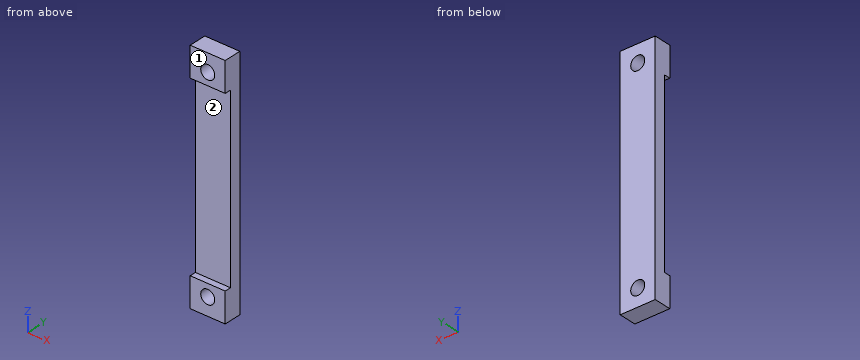
Autodesk Inventor part; units mm, degrees
ref_plane "YZ Plane" through (0, 0, 0) normal (1, 0, 0) x (0, 1, 0)
ref_plane "XZ Plane" through (0, 0, 0) normal (0, 1, 0) x (-1, 0, 0)
ref_plane "XY Plane" through (0, 0, 0) normal (0, 0, 1) x (1, 0, 0)
sketch "Эскиз1" plane through (0, 0, 0) normal (0, 1, 0) x (-1, 0, 0)
  line L0 (-8, -25.5) -> (-10, -25.5)
  line L1 (-10, -34) -> (-10, -25.5)
  line L2 (0, -34) -> (-10, -34)
  line L3 (0, -34) -> (0, -25.5)
  line L4 (0, -25.5) -> (-2, -25.5)
  line L5 (-2, -25.5) -> (-2, 25.5)
  line L6 (-2, 25.5) -> (0, 25.5)
  line L7 (0, 25.5) -> (0, 34)
  line L8 (0, 34) -> (-10, 34)
  line L9 (-10, 25.5) -> (-10, 34)
  line L10 (-10, 25.5) -> (-8, 25.5)
  line L11 (-8, 25.5) -> (-8, -25.5)
  line L12 (-4, 25.5) -> (-4, -25.5)
  line L13 (-4, -25.5) -> (-6, -25.5)
  line L14 (-6, -25.5) -> (-6, 25.5)
  line L15 (-6, 25.5) -> (-4, 25.5)
  circle A0 centre (-5, 29) radius 2
  circle A1 centre (-5, -29) radius 2
  line L16 (-10, 25.5) -> (-10, -25.5)
  line L17 (-10, -25.5) -> (-8, -25.5)
  line L18 (-8, -25.5) -> (-8, 25.5)
  line L19 (-8, 25.5) -> (-10, 25.5)
  line L20 (0, 25.5) -> (-2, 25.5)
  line L21 (-2, 25.5) -> (-2, -25.5)
  line L22 (-2, -25.5) -> (0, -25.5)
  line L23 (0, -25.5) -> (0, 25.5)
  point P0 (0, 0)
  point P1 (0, 0)
extrude "Выдавливание1" add sketch "Эскиз1" along normal blind 5 contours L11 L10 L9 L8 L7 L6 L5 L4 L3 L2 L1 L0 | L0 L16 L10 L11 | L4 L5 L6 L23 | L12 L13 L14 L15
sketch "Эскиз2" plane through (0, 0, 0) normal (0, -1, 0) x (1, 0, 0)
  line L0 (10, 34) -> (10, -34)
  line L1 (10, 0) -> (0, 0)
  line L2 (0, -34) -> (0, 34)
  line L3 (0, 25.5) -> (10, 25.5)
  line L4 (10, 25.5) -> (10, -25.5)
  line L5 (10, -25.5) -> (0, -25.5)
  line L6 (0, -25.5) -> (0, 25.5)
  line L7 (0, 25.5) -> (10, -25.5) construction
  line L8 (10, 25.5) -> (0, -25.5) construction
  point P0 (5, 0)
  dimension "d2" = 51
extrude "Выдавливание2" cut sketch "Эскиз2" against normal blind 1.8
properties part number "КВ33.044.305 - Прижим ремня" material "Пластик АБС"
Could you check a few things on this model? Use its own coordinates, in mm. Face numbers are marked on the shaded views. Coordinates: 2 decimals unless noted, no trailing zeros. Order: outer loops, then holes, each group sorted by start corner. A loop starts at its lowest first (then second) coordinate and runs counter-clockwise, first axis right, second up. Notation, with made-up numbers: (-30.75, 3.25) -> (8.25, 3.25) arc R31 ccw to (8.25, 38.25) -> close; hole circle Ø8 at (29, 58.5). An arc over 180 degrees is marked (long way). One line per question, with ' | ' between items.
Q1. Thinking about a two-plate mould opening in Z: for the marked faces 1 and 2, which applies, pulls with the +Z half, pulls with the -Z half, needs draft (parallel to the pull), parting line crosses it, or undercut?
Return value:
face 1: needs draft | face 2: undercut
Q2. I'm going to push a flat-ended pin straight in: P1, Ø3, axis at x = 4.5, z = 11.5, coming from the -Y side. Where does the tip first touch, or does it pass through?
Return value:
P1: y = 1.8
Q3. If I drill on L1, parallel to Z at x = 5, y = 3.05; L2, parallel to Z at x = 5, y = 1.7; L3, parallel to Z at x = 1, y = 0.55, over which ranges is the centre line in solid material (lowest first)?
Return value:
L1: -34 to -31, -27 to 27, 31 to 34 | L2: -34 to -31, -27 to -25.5, 25.5 to 27, 31 to 34 | L3: -34 to -25.5, 25.5 to 34
Q4. Imagine slicing it at A-A on y = 0.9. Please give me the cut outline in (x, z).
Return value:
outline: (0, -34) -> (10, -34) -> (10, -25.5) -> (0, -25.5) -> close; (0, 25.5) -> (10, 25.5) -> (10, 34) -> (0, 34) -> close; hole circle Ø4 at (5, -29); hole circle Ø4 at (5, 29)
Q5. Imagine slicing it at D-D on y = 3.6. Please give me the cut outline in (x, z), and give its area (3 significant figures).
Return value:
outline: (0, -34) -> (10, -34) -> (10, 34) -> (0, 34) -> close; hole circle Ø4 at (5, -29); hole circle Ø4 at (5, 29) | area: 655 mm²
Q6. Imagine slicing it at C-C on z = 29. Please give me the cut outline in (x, y).
Return value:
outline: (0, 0) -> (3, 0) -> (3, 5) -> (0, 5) -> close; (7, 0) -> (10, 0) -> (10, 5) -> (7, 5) -> close
Q7. Imagine slicing it at B-B on x = 5. Please give me the cut outline in (y, z), and give its area (3 significant figures).
Return value:
outline: (0, -34) -> (5, -34) -> (5, -31) -> (0, -31) -> close; (0, -27) -> (5, -27) -> (5, 27) -> (0, 27) -> (0, 25.5) -> (1.8, 25.5) -> (1.8, -25.5) -> (0, -25.5) -> close; (0, 31) -> (5, 31) -> (5, 34) -> (0, 34) -> close | area: 208 mm²
